from build123d import *

# Parameters (mm, degrees)
REVOLVE1_ANGLE      = 270
BOSS_EXTRUDE1_DEPTH = 50
SKETCH3_R           = 12.5
CUT_EXTRUDE2_DEPTH  = 51


with BuildPart() as part:
    # Sketch1 → Revolve1 (revolve)
    with BuildSketch(Plane(origin=(0, 0, 0), x_dir=(1, 0, 0), z_dir=(0, 1, 0))):
        with BuildLine():
            Line((15, 50), (25, 50))
            Line((25, 50), (25, 0))
            Line((25, 0), (-25, 0))
            Line((-25, 0), (-25, 50))
            Line((-25, 50), (-15, 50))
            ThreePointArc((-15, 50), (0, 35), (15, 50))
        make_face()
    revolve(axis=Axis((-25, 0, 0), (1, 0, 0)), revolution_arc=REVOLVE1_ANGLE)

    # Sketch1<2> → Boss-Extrude1 (add)
    with BuildSketch(Plane(origin=(0, 0, 0), x_dir=(1, 0, 0), z_dir=(0, 1, 0))):
        with BuildLine():
            Line((15, 50), (25, 50))
            Line((25, 50), (25, 0))
            Line((25, 0), (-25, 0))
            Line((-25, 0), (-25, 50))
            Line((-25, 50), (-15, 50))
            ThreePointArc((-15, 50), (0, 35), (15, 50))
        make_face()
    extrude(amount=-BOSS_EXTRUDE1_DEPTH)

    # Sketch3 → Cut-Extrude2 (cut, through all)
    with BuildSketch(Plane(origin=(25, 0, 0), x_dir=(0, 0, -1), z_dir=(1, 0, 0))):
        Circle(SKETCH3_R)
    extrude(amount=-CUT_EXTRUDE2_DEPTH, mode=Mode.SUBTRACT)


solid = part.part
Build history of the part. All positions in model axes, mm. Round coordinates to 2 decimals unless told otherwise and drop trailing zeros. Write each loop counter-clockwise with the first axis right and the second up, starting at its lowest first coordinate (ties: lowest second). Pieces come first, ordered by that corner, then holes. Notation, with made-up numbers: (51.5, 38.5) -> (103.5, 38.5) arc R14 ccw to (103.5, 42.5) -> close; hole circle Ø9 at (15, -9.75). An arc over 180 degrees is marked (long way). Use one line per item in the form item = value.
Q1. Drop flat-ended pins along their axis: P1, Ø5, axis at x = -17, y = 13.5, coming from the +Z side (3 decimals); P2, Ø16.5, axis at x = 5, y = -46, coming from the +Z side; P3, Ø8, axis at x = -9.5, z = 12.5, coming from the +Y side. Give the stop position or say it passes through.
Conclusion:
P1 = 48.775
P2 = 0
P3 = 41.71
Q2. Drill centre lines: L1, parallel to X at y = 30, z = -39; L2, parallel to X at y = -0.5, z = -36.5; L3, parallel to Y at x = -10, z = 11. Where is each one in solid material? Low to high.
Conclusion:
L1 = -25 to -14.98, 14.98 to 25
L2 = -25 to -6.54, 6.54 to 25
L3 = -37.23 to -5.94, 5.94 to 37.23
Q3. Two-plate mould, pull along Z, no slides. Class faces 1 (the cylindrical face through (0.35, 3.755, -11.923)), 2 (the flat face through (-20, -25, -50)), 3 (the flat face through (0, -44, 0)): released by +Z, released by -Z, zero draft, split by the parting line, or undercut.
Conclusion:
face_1 = undercut
face_2 = released by -Z
face_3 = released by +Z
Q4. Band-saw the part on C-C, the plane x = 8. Write the cut outline in (y, z), then the cut area to 3 significant figures.
Conclusion:
outline = (-50, -37.31) -> (0, -37.31) arc R37.31 ccw (long way) to (-37.31, 0) -> (-50, 0) -> close; hole circle Ø25 at (0, 0)
area = 4,650 mm²
Q5. Band-saw the part on B-B, the plane x = -17. Write the cut outline in (y, z).
Conclusion:
outline = (-50, -50) -> (0, -50) arc R50 ccw (long way) to (-50, 0) -> close; hole circle Ø25 at (0, 0)
Q6. Band-saw the part on A-A, the plane x = 0. Write the cut outline in (y, z), then the cut area to 3 significant figures.
Conclusion:
outline = (-50, -35) -> (0, -35) arc R35 ccw (long way) to (-35, 0) -> (-50, 0) -> close; hole circle Ø25 at (0, 0)
area = 4,150 mm²
